```python
from build123d import *

# Parameters (mm, degrees)
F0_R      = 44.4398
F1_DEPTH  = 94.996
F2_W      = 121.819742
F2_H      = 87.529742
F3_DEPTH  = 19.304
F4_R      = 38.081956
F5_DEPTH  = 37.084
F6_R      = 15.067271
F7_DEPTH  = 25.4
F8_R      = 27.350413
F9_DEPTH  = 8.636
F10_R     = 38.756929
F11_DEPTH = 20.32
F12_W     = 14.738686
F12_H     = 87.529742
F13_DEPTH = 25.4


with BuildPart() as f1:
    # F0 (on Top) → F1 (new body)
    with BuildSketch(Plane.XY):
        with Locations((2.556712, 0)):
            Circle(F0_R)
    extrude(amount=F1_DEPTH)

    # F2 (on face) → F3 (join)
    with BuildSketch(Plane(origin=(0, 0, 0), x_dir=(1, 0, 0), z_dir=(0, 0, -1))):
        Rectangle(F2_W, F2_H)
    extrude(amount=F3_DEPTH)

    # F4 (on face) → F5 (join)
    with BuildSketch(Plane(origin=(0, 0, -19.304), x_dir=(1, 0, 0), z_dir=(0, 0, -1))):
        with Locations((15.189868, 0)):
            Circle(F4_R)
    extrude(amount=F5_DEPTH)

    # F6 (on face) → F7 (join)
    with BuildSketch(Plane(origin=(0, 0, -56.388), x_dir=(1, 0, 0), z_dir=(0, 0, -1))):
        with Locations((22.709604, 0)):
            Circle(F6_R)
    extrude(amount=F7_DEPTH)

    # F8 (on face) → F9 (join)
    with BuildSketch(Plane.XY.offset(94.996)):
        Circle(F8_R)
    extrude(amount=F9_DEPTH)

    # F10 (on face) → F11 (join)
    with BuildSketch(Plane.XY.offset(103.632)):
        Circle(F10_R)
    extrude(amount=F11_DEPTH)

    # F12 (on face) → F13 (join)
    with BuildSketch(Plane.XY):
        with Locations((-53.540528, 0)):
            Rectangle(F12_W, F12_H)
    extrude(amount=F13_DEPTH)


solid = f1.part
```
Part model, mm, in its own coordinate system. A direction names the side the tool comes from. Round coordinates to 2 decimals unless told otherwise and drop trailing zeros. Write each loop counter-clockwise with the first axis right and the second up, starting at its lowest first coordinate (ties: lowest second). Pieces come first, ordered by that corner, then holes.
Item 1: Drop flat-ended pins along their axis: pin 1 Ø1.5 at (x, z) = (-15.5, -47.5) entering from +Y; pin 2 Ø10 at (x, y) = (-34.5, -33) entering from +Z; pin 3 Ø23.5 at (x, y) = (1, 18) entering from -Z. Give the stop position or say it passes through.
Results:
pin 1: stops at y = 23.53
pin 2: stops at z = 0
pin 3: stops at z = -56.39
Item 2: Probe L1, parallel to Z at x = -28.5, y = -20; L2, parallel to Z at x = 28, y = -25; L3, parallel to Z at x = -37, y = 23. List the from-to ranges inside material, lowest first.
Results:
L1: z = -19.3 to 95, 103.63 to 123.95
L2: z = -56.39 to 95, 103.63 to 123.95
L3: z = -19.3 to 0
Item 3: Cut at C-C, the plane x = 0. Give the cut face in (y, z), plus the area to 3 significant figures.
Results:
outline: (-44.37, 0) - (-43.76, 0) - (-43.76, -19.3) - (-34.92, -19.3) - (-34.92, -56.39) - (34.92, -56.39) - (34.92, -19.3) - (43.76, -19.3) - (43.76, 0) - (44.37, 0) - (44.37, 95) - (27.35, 95) - (27.35, 103.63) - (38.76, 103.63) - (38.76, 123.95) - (-38.76, 123.95) - (-38.76, 103.63) - (-27.35, 103.63) - (-27.35, 95) - (-44.37, 95) - close
area: 14,800 mm2
Item 4: Cut at D-D, the plane y = 0. Give the cut face in (x, z).
Results:
outline: (-60.91, -19.3) - (-22.89, -19.3) - (-22.89, -56.39) - (7.64, -56.39) - (7.64, -81.79) - (37.78, -81.79) - (37.78, -56.39) - (53.27, -56.39) - (53.27, -19.3) - (60.91, -19.3) - (60.91, 0) - (47, 0) - (47, 95) - (27.35, 95) - (27.35, 103.63) - (38.76, 103.63) - (38.76, 123.95) - (-38.76, 123.95) - (-38.76, 103.63) - (-27.35, 103.63) - (-27.35, 95) - (-41.88, 95) - (-41.88, 0) - (-46.17, 0) - (-46.17, 25.4) - (-60.91, 25.4) - close
Item 5: Two-plate mould, pull along Z, no slides. Class faces 1 (the flat face through (22, -19, 94.996)), 2 (the flat face through (-1, -43.765, -7)), 3 (the cylindrical face through (26.087, 8.215, 99.254)), 4 (the flat face through (-42, 3, 0)): +Z half, -Z half, draft (parallel to the pull), parting line (faces both ways), or undercut.
Results:
face 1: undercut
face 2: draft
face 3: undercut
face 4: +Z half
Item 6: Cut at B-B, the plane y = 35. Give the cut face in (x, z).
Results:
outline: (-60.91, -19.3) - (0.18, -19.3) - (0.18, -56.39) - (30.2, -56.39) - (30.2, -19.3) - (60.91, -19.3) - (60.91, 0) - (29.94, 0) - (29.94, 95) - (-24.83, 95) - (-24.83, 0) - (-46.17, 0) - (-46.17, 25.4) - (-60.91, 25.4) - close; (-16.65, 103.63) - (16.65, 103.63) - (16.65, 123.95) - (-16.65, 123.95) - close
Item 7: Cut at A-A, the plane z = 22. Give the cut face in (x, y), plus the area to 3 significant figures.
Results:
outline: (-60.91, -43.76) - (-46.17, -43.76) - (-46.17, 43.76) - (-60.91, 43.76) - close; circle Ø88.88 at (2.56, 0)
area: 7,490 mm2
Item 8: Which spindle directions (+Z, -Z, +X, -X, +Y, -Y) get a long thin tool onto all of the face, cutting with end or side? Do faces 5 (the flat face through (-46.171, -1, 13)), 6 (the flat face through (-28, -1, -19.304)), 7 (the flat face through (-54, 1, 25.4)), 8 (the cylindrical face through (-8.402, -37.835, 113.65)). Say none if no direction does.
Results:
face 5: +Z, +Y, -Y
face 6: -Z
face 7: +Z, -X, +Y, -Y
face 8: +Z
